```python
from build123d import *

# Parameters (mm, degrees)
SKETCH_1_W      = 15
SKETCH_1_H      = 32
EXTRUDE_1_DEPTH = 1.6
SKETCH_2_W      = 12.857079129
SKETCH_2_H      = 21.128766401
EXTRUDE_2_DEPTH = 2
SKETCH_3_R      = 1.048746982
EXTRUDE_3_DEPTH = 1.8


with BuildPart() as part:
    # 草图1 → 凸台-拉伸1 (new body)
    with BuildSketch(Plane(origin=(0, 0, 0), x_dir=(1, 0, 0), z_dir=(0, 1, 0))):
        Rectangle(SKETCH_1_W, SKETCH_1_H)
    extrude(amount=EXTRUDE_1_DEPTH)

    # 草图2 → 凸台-拉伸2 (add)
    with BuildSketch(Plane(origin=(0, 1.6, 0), x_dir=(1, 0, 0), z_dir=(0, 1, 0))):
        with Locations((0.002075323, -4.405572569)):
            Rectangle(SKETCH_2_W, SKETCH_2_H)
    extrude(amount=EXTRUDE_2_DEPTH)

    # 草图3 → 凸台-拉伸3 (add)
    with BuildSketch(Plane(origin=(0, 1.6, 0), x_dir=(1, 0, 0), z_dir=(0, 1, 0))):
        with Locations(Location((-5.062783927, 12.209984483, 0), (0, 0, 270))):
            Circle(SKETCH_3_R)
    extrude(amount=EXTRUDE_3_DEPTH)


solid = part.part
```
Can you work these out from the model? Positions are in its coordinate system, mm. A direction names the side the tool comes from. Coordinates: 2 decimals unless noted, no trailing zeros. Loops run counter-clockwise (first coordinate to the right, second up) from the corner with the lowest first, then second, coordinate; pieces in that order, holes last. Notation, with made-up numbers: (19, 10.25) -> (38, 10.25) arc R20 cw to (38, 32.25) -> close; hole circle Ø6 at (33, -27.5). An arc over 180 degrees is marked (long way). Answer as a JSON object with one key per item and string values.
1) For P1, Ø2, axis at x = -5, y = 2.5, coming from the -Z side; P2, Ø1.6, axis at x = -2.5, y = 2.5, coming from the -Z side; P3, Ø1, axis at x = -0.5, z = -12, coming from the +Y side; P4, Ø0.6, axis at x = 0, y = 2.5, coming from the +Z side, each with a flat end and sliding along its axis, tell me the tip position at first contact or that it passes through.
Results:
{"P1": "stops at z = -16", "P2": "stops at z = -6.16", "P3": "stops at y = 1.6", "P4": "stops at z = 14.97"}
2) Imagine slicing it at A-A (y = 2.25). Please give me the cut outline in (x, z), then the cut area to 3 significant figures.
Results:
{"outline": "(-6.43, -6.16) -> (6.43, -6.16) -> (6.43, 14.97) -> (-6.43, 14.97) -> close; circle Ø2.1 at (-5.06, -12.21)", "area": "275 mm^2"}
3) For faces 1 (the face through (6.431, 3, 5)), 2 (the face through (-5, 3.4, -12)), 3 (the face through (0, 3, 14.97)), 4 (the face through (0, 3, -6.159)), 5 (the face through (-6.426, 3, 5)), which set-ups out of +Z, -Z, +X, -X, +Y, -Y let a thin tool reach every point of the face, with its end or its side?
Results:
{"face 1": "+Z, -Z, +X, +Y", "face 2": "-Z, +X, -X, +Y", "face 3": "+Z, +X, -X, +Y", "face 4": "+X, -X, +Y", "face 5": "+Z, -Z, -X, +Y"}
4) If I drill on line 1 (X direction, y = 1.85, z = -1); line 2 (Z direction, x = 1.25, y = 2.9); line 3 (Y direction, x = 6.5, z = -10), over which ranges is the centre line in solid material (lowest first)?
Results:
{"line 1": "x = -6.43 to 6.43", "line 2": "z = -6.16 to 14.97", "line 3": "y = 0 to 1.6"}
5) Imagine slicing it at C-C (x = 5.25). Please give me the cut outline in (y, z), then the cut area to 3 significant figures.
Results:
{"outline": "(0, -16) -> (1.6, -16) -> (1.6, -6.16) -> (3.6, -6.16) -> (3.6, 14.97) -> (1.6, 14.97) -> (1.6, 16) -> (0, 16) -> close", "area": "93.5 mm^2"}
6) Imagine slicing it at B-B (z = -3). Please give me the cut outline in (x, y), then the cut area to 3 significant figures.
Results:
{"outline": "(-7.5, 0) -> (7.5, 0) -> (7.5, 1.6) -> (6.43, 1.6) -> (6.43, 3.6) -> (-6.43, 3.6) -> (-6.43, 1.6) -> (-7.5, 1.6) -> close", "area": "49.7 mm^2"}
7) Thinking about a two-plate mould opening in Z: for faces 6 (the face through (0, 0, 0)), 7 (the face through (-4.35, 2.49, -12.98)), 8 (the face through (0, 1, -16)), which applies, pulls with the +Z half, pulls with the -Z half, needs draft (parallel to the pull), parting line crosses it, or undercut?
Results:
{"face 6": "needs draft", "face 7": "undercut", "face 8": "pulls with the -Z half"}
8) Imagine slicing it at D-D (z = -6.5). Please give me the cut outline in (x, y).
Results:
{"outline": "(-7.5, 0) -> (7.5, 0) -> (7.5, 1.6) -> (-7.5, 1.6) -> close"}
